Geometry: final body of the model. Coordinates: model frame, mm. Face numbers are marked on the shaded views. A direction names the side the tool comes from. Give positions to 0.01 mm unless a question says otherwise; leave off trailing zeros. Write each loop counter-clockwise with the first axis right and the second up, starting at its lowest first coordinate (ties: lowest second). Pieces come first, ordered by that corner, then holes.
```python
from build123d import *

# Parameters (mm, degrees)
F1_DEPTH = 25.4
F2_R     = 42.411309
F3_DEPTH = 25.4


with BuildPart() as f1:
    # F0 (on Top) → F1 (new body)
    with BuildSketch(Plane.XY):
        Polygon((19.05, 72.694803), (-72.694803, 19.05), (-19.05, -72.694803), (72.694803, -19.05), align=None)
    extrude(amount=F1_DEPTH)

    # F2 (on face) → F3 (join)
    with BuildSketch(Plane.XY.offset(25.4)):
        Circle(F2_R)
    extrude(amount=F3_DEPTH)

    # F4 (on face) → F5 (revolve)
    with BuildSketch(Plane.XY.offset(50.8)):
        with BuildLine():
            Line((0, 27.8892), (0, -27.8892))
            ThreePointArc((0, -27.8892), (27.8892, 0), (0, 27.8892))
        make_face()
    revolve(axis=Axis((0, 0, 50.8), (0, -1, 0)))


solid = f1.part
```
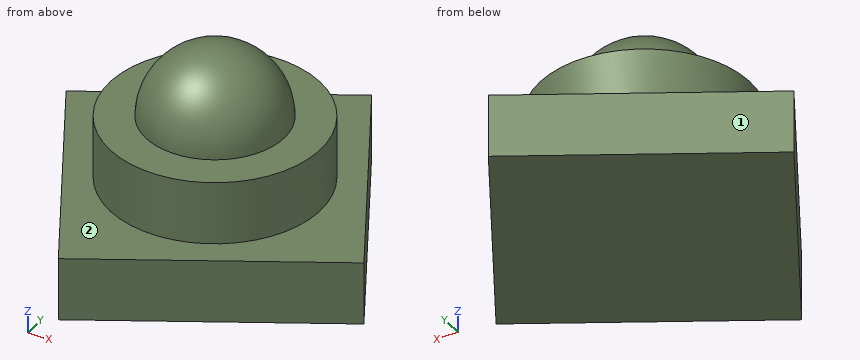
Item 1: Section C-C, the plane z = 48. Return the cut outline in (x, y), plus the area to 3 significant figures.
Found:
outline: circle Ø84.82 at (0, 0)
area: 5,650 mm2
Item 2: Pin query (flat end, axial travel): pin 1 Ø1.5 at (x, z) = (-15, 27.5) entering from -Y; pin 2 Ø5 at (y, z) = (-10, 25) entering from -X; pin 3 Ø5 at (x, z) = (29.5, 48.5) entering from +Y. Return the tip coordinate at first contact, or that it passes through.
Found:
pin 1: stops at y = -39.95
pin 2: stops at x = -57.17
pin 3: stops at y = 32.71
Item 3: Section A-A, the plane y = 0. Return the cut outline in (x, z), plus the area to 3 significant figures.
Found:
outline: (-61.56, 0) - (61.56, 0) - (61.56, 25.4) - (42.41, 25.4) - (42.41, 50.8) - (27.89, 50.8) arc R27.89 ccw to (-27.89, 50.8) - (-42.41, 50.8) - (-42.41, 25.4) - (-61.56, 25.4) - close
area: 6,500 mm2
Item 4: Reachability of the marked faces 1 and 2 from +Z, -Z, +X, -X, +Y, -Y: full face, straight path, thin tool, end or side. Return the list, or none.
Found:
face 1: +Z, -Z, -X, +Y
face 2: +Z
Item 5: Line query: L1, parallel to Z at x = -7, y = -47.5; L2, parallel to Z at x = 2, y = 28; L3, parallel to Y at x = -0.5, z = 17. Output: solid intervals per line, ascending.
Found:
L1: z = 0 to 25.4
L2: z = 0 to 50.8
L3: y = -61.85 to 61.26
Item 6: Section D-D, the plane x = -33.5. Return the cut outline in (y, z).
Found:
outline: (-47.98, 0) - (41.97, 0) - (41.97, 25.4) - (26.01, 25.4) - (26.01, 50.8) - (-26.01, 50.8) - (-26.01, 25.4) - (-47.98, 25.4) - close
Item 7: Section B-B, the plane x = -9.5. Return the cut outline in (y, z).
Found:
outline: (-67.11, 0) - (56, 0) - (56, 25.4) - (41.33, 25.4) - (41.33, 50.8) - (26.22, 50.8) arc R26.22 ccw to (-26.22, 50.8) - (-41.33, 50.8) - (-41.33, 25.4) - (-67.11, 25.4) - close
